Geometry: final body of the model. Coordinates: model frame, mm. Give positions to 0.01 mm unless a question says otherwise; leave off trailing zeros. Loops run counter-clockwise (first coordinate to the right, second up) from the corner with the lowest first, then second, coordinate; pieces in that order, holes last. Notation, with made-up numbers: (88.5, 4) -> (145.5, 4) arc R22 ccw to (145.5, 33) -> close; hole circle Ø5 at (9.25, 80). An arc over 180 degrees is marked (long way). One line per question, with ' | ' between items. Start each with the question number.
Item 1: Section A-A on x = 10. Return loops of the section in (y, z), then the cut area to 3 significant figures.
Item 2: Section B-B on y = -7.9. Return loops of the section in (x, z).
Item 3: Section C-C on z = -0.9. Return loops of the section in (x, y).
Item 4: Section D-D on x = -3.75. Return loops of the section in (y, z).
Item 5: Material intervals for line 1 along X through (y, z) = (5.5, 0.25); line 2 along Z through (x, y) = (-8.5, 0); line 3 along X through (y, z) = (8, -1.05), sorted ascending. Write a range as [from, to].
Item 6: Pin query (flat end, axial travel): P1, Ø0.5, axis at x = -10.5, z = 0.5, coming from the +Y side; P2, Ø8, axis at x = 3.5, y = -2, coming from the -Z side; P3, Ø0.7, axis at y = 10.5, z = 0, coming from the +X side; P4, Ø1.2, axis at x = 0, y = 0, coming from the +Z side. Return the tip coordinate at first contact, or that it passes through.
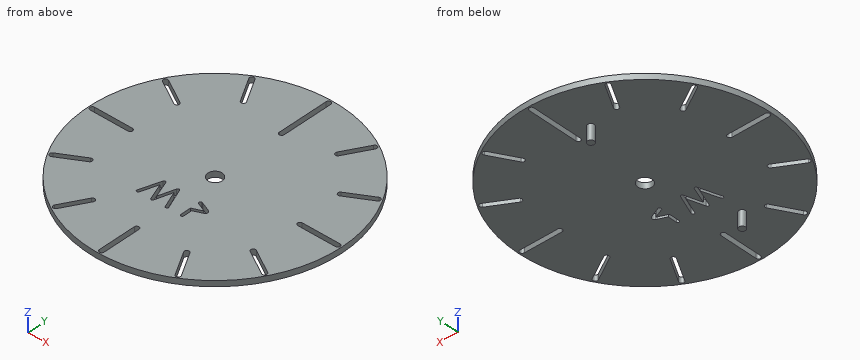
from build123d import *

# Parameters (mm, degrees)
F0_R     = 13.375
F1_DEPTH = 0.6
F2_R     = 0.75
F3_DEPTH = 0.6
F4_R     = 0.35
F5_DEPTH = 2.2


with BuildPart() as f1:
    # F0 (on Top) → F1 (new body)
    with BuildSketch(Plane.XY):
        Circle(F0_R)
        with BuildLine():
            Line((-2.455603, -3.641186), (-3.03039, -5.425586))
            ThreePointArc((-3.03039, -5.425586), (-3.219156, -5.522371), (-3.315941, -5.333605))
            Line((-3.315941, -5.333605), (-2.609415, -3.140224))
            ThreePointArc((-2.609415, -3.140224), (-2.470382, -3.036261), (-2.326336, -3.133157))
            Line((-2.326336, -3.133157), (-1.656765, -4.903756))
            Line((-1.656765, -4.903756), (-1.138734, -3.161121))
            ThreePointArc((-1.138734, -3.161121), (-1.00206, -3.054032), (-0.855862, -3.147702))
            Line((-0.855862, -3.147702), (0.01888, -5.31412))
            ThreePointArc((0.01888, -5.31412), (-0.064049, -5.50937), (-0.2593, -5.426441))
            Line((-0.2593, -5.426441), (-0.973416, -3.657835))
            Line((-0.973416, -3.657835), (-1.487491, -5.387162))
            ThreePointArc((-1.487491, -5.387162), (-1.615532, -5.529433), (-1.78089, -5.433038))
            Line((-1.78089, -5.433038), (-2.455603, -3.641186))
        make_face(mode=Mode.SUBTRACT)
        with BuildLine():
            ThreePointArc((1.625497, -5.364779), (1.475497, -5.514779), (1.325497, -5.364779))
            Line((1.325497, -5.364779), (1.325497, -4.433364))
            Line((1.325497, -4.433364), (1.325497, -4.248424))
            Line((1.325497, -4.248424), (2.363726, -3.807202))
            Line((2.363726, -3.807202), (1.325497, -3.371863))
            ThreePointArc((1.325497, -3.371863), (1.302815, -3.187375), (1.450294, -3.074238))
            Line((1.450294, -3.074238), (1.625497, -3.147702))
            Line((1.625497, -3.147702), (2.61069, -3.560803))
            ThreePointArc((2.61069, -3.560803), (2.724561, -3.786736), (2.612869, -4.013755))
            Line((2.612869, -4.013755), (2.483792, -4.068609))
            Line((2.483792, -4.068609), (1.625497, -4.433364))
            Line((1.625497, -4.433364), (1.625497, -5.364779))
        make_face(mode=Mode.SUBTRACT)
    extrude(amount=F1_DEPTH)

    # F2 (on face) → F3 (cut, through all)
    with BuildSketch(Plane.XY.offset(0.6)):
        with BuildLine():
            ThreePointArc((-11.121827, 6.709865), (-11.463333, 6.618359), (-11.371827, 6.276852))
            Line((-11.371827, 6.276852), (-8.773751, 4.776852))
            ThreePointArc((-8.773751, 4.776852), (-8.432244, 4.868359), (-8.523751, 5.209865))
            Line((-8.523751, 5.209865), (-11.121827, 6.709865))
        make_face()
        with BuildLine():
            Line((-8.986717, 0.25), (-12.986717, 0.25))
            ThreePointArc((-12.986717, 0.25), (-13.236717, 0), (-12.986717, -0.25))
            Line((-12.986717, -0.25), (-8.986717, -0.25))
            ThreePointArc((-8.986717, -0.25), (-8.736717, 0), (-8.986717, 0.25))
        make_face()
        with BuildLine():
            ThreePointArc((-6.276852, 11.371827), (-6.618359, 11.463333), (-6.709865, 11.121827))
            Line((-6.709865, 11.121827), (-5.209865, 8.523751))
            ThreePointArc((-5.209865, 8.523751), (-4.868359, 8.432244), (-4.776852, 8.773751))
            Line((-4.776852, 8.773751), (-6.276852, 11.371827))
        make_face()
        with BuildLine():
            ThreePointArc((-0.25, 8.986717), (-0.176777, 9.163494), (0, 9.236717))
            ThreePointArc((0, 9.236717), (0.176777, 9.163494), (0.25, 8.986717))
            Line((0.25, 8.986717), (0.25, 12.986717))
            ThreePointArc((0.25, 12.986717), (0, 13.236717), (-0.25, 12.986717))
            Line((-0.25, 12.986717), (-0.25, 8.986717))
        make_face()
        with BuildLine():
            ThreePointArc((6.709865, 11.121827), (6.618359, 11.463333), (6.276852, 11.371827))
            Line((6.276852, 11.371827), (4.776852, 8.773751))
            ThreePointArc((4.776852, 8.773751), (4.868359, 8.432244), (5.209865, 8.523751))
            Line((5.209865, 8.523751), (6.709865, 11.121827))
        make_face()
        with BuildLine():
            ThreePointArc((11.371827, 6.276852), (11.463333, 6.618359), (11.121827, 6.709865))
            Line((11.121827, 6.709865), (8.523751, 5.209865))
            ThreePointArc((8.523751, 5.209865), (8.432244, 4.868359), (8.773751, 4.776852))
            Line((8.773751, 4.776852), (11.371827, 6.276852))
        make_face()
        with BuildLine():
            Line((8.986717, -0.25), (12.986717, -0.25))
            ThreePointArc((12.986717, -0.25), (13.236717, 0), (12.986717, 0.25))
            Line((12.986717, 0.25), (8.986717, 0.25))
            ThreePointArc((8.986717, 0.25), (8.736717, 0), (8.986717, -0.25))
        make_face()
        with BuildLine():
            ThreePointArc((11.121827, -6.709865), (11.463333, -6.618359), (11.371827, -6.276852))
            Line((11.371827, -6.276852), (8.773751, -4.776852))
            ThreePointArc((8.773751, -4.776852), (8.432244, -4.868359), (8.523751, -5.209865))
            Line((8.523751, -5.209865), (11.121827, -6.709865))
        make_face()
        with BuildLine():
            Line((-0.25, -8.986717), (-0.25, -12.986717))
            ThreePointArc((-0.25, -12.986717), (0, -13.236717), (0.25, -12.986717))
            Line((0.25, -12.986717), (0.25, -8.986717))
            ThreePointArc((0.25, -8.986717), (0, -8.736717), (-0.25, -8.986717))
        make_face()
        with BuildLine():
            ThreePointArc((6.276852, -11.371827), (6.618359, -11.463333), (6.709865, -11.121827))
            Line((6.709865, -11.121827), (5.209865, -8.523751))
            ThreePointArc((5.209865, -8.523751), (4.868359, -8.432244), (4.776852, -8.773751))
            Line((4.776852, -8.773751), (6.276852, -11.371827))
        make_face()
        with BuildLine():
            ThreePointArc((-6.709865, -11.121827), (-6.618359, -11.463333), (-6.276852, -11.371827))
            Line((-6.276852, -11.371827), (-4.776852, -8.773751))
            ThreePointArc((-4.776852, -8.773751), (-4.868359, -8.432244), (-5.209865, -8.523751))
            Line((-5.209865, -8.523751), (-6.709865, -11.121827))
        make_face()
        with BuildLine():
            ThreePointArc((-11.371827, -6.276852), (-11.463333, -6.618359), (-11.121827, -6.709865))
            Line((-11.121827, -6.709865), (-8.523751, -5.209865))
            ThreePointArc((-8.523751, -5.209865), (-8.432244, -4.868359), (-8.773751, -4.776852))
            Line((-8.773751, -4.776852), (-11.371827, -6.276852))
        make_face()
        Circle(F2_R)
        with BuildLine():
            ThreePointArc((0, 8.736717), (-0.176777, 8.80994), (-0.25, 8.986717))
            Line((-0.25, 8.986717), (-0.25, 7.62564))
            ThreePointArc((-0.25, 7.62564), (0, 7.37564), (0.25, 7.62564))
            Line((0.25, 7.62564), (0.25, 8.986717))
            ThreePointArc((0.25, 8.986717), (0.176777, 8.80994), (0, 8.736717))
        make_face()
        with BuildLine():
            Line((0, 8.986717), (0, 9.236717))
            ThreePointArc((0, 9.236717), (-0.176777, 9.163494), (-0.25, 8.986717))
            ThreePointArc((-0.25, 8.986717), (-0.176777, 8.80994), (0, 8.736717))
            Line((0, 8.736717), (0, 8.986717))
        make_face()
        with BuildLine():
            ThreePointArc((0.25, 8.986717), (0.176777, 9.163494), (0, 9.236717))
            Line((0, 9.236717), (0, 8.986717))
            Line((0, 8.986717), (0, 8.736717))
            ThreePointArc((0, 8.736717), (0.176777, 8.80994), (0.25, 8.986717))
        make_face()
    extrude(amount=-F3_DEPTH, mode=Mode.SUBTRACT)

    # F4 (on face) → F5 (join)
    with BuildSketch(Plane.XY.offset(0.6)):
        with Locations((-1.9, 8.234)):
            Circle(F4_R)
        with Locations((-3, -7.9)):
            Circle(F4_R)
    extrude(amount=-F5_DEPTH)


solid = f1.part
Result sheet:
1) outline: (-8.88, 0) -> (-6.06, 0) -> (-6.06, 0.6) -> (-8.88, 0.6) -> close; (-5.48, 0) -> (-0.25, 0) -> (-0.25, 0.6) -> (-5.48, 0.6) -> close; (0.25, 0) -> (5.48, 0) -> (5.48, 0.6) -> (0.25, 0.6) -> close; (6.06, 0) -> (8.88, 0) -> (8.88, 0.6) -> (6.06, 0.6) -> close | area: 9.67 mm²
2) outline: (-10.79, 0) -> (-3.35, 0) -> (-3.35, -1.6) -> (-2.65, -1.6) -> (-2.65, 0) -> (10.79, 0) -> (10.79, 0.6) -> (-10.79, 0.6) -> close
3) outline: circle Ø0.7 at (-3, -7.9); circle Ø0.7 at (-1.9, 8.23)
4) outline: (-12.84, 0) -> (12.84, 0) -> (12.84, 0.6) -> (-12.84, 0.6) -> close
5) line 1: x = [-12.19, -10.03], [-9.03, 9.03], [10.03, 12.19] | line 2: z = [0, 0.6] | line 3: x = [-2.16, -1.64]
6) P1: stops at y = 8.59 | P2: stops at z = 0 | P3: stops at x = 8.71 | P4: passes through
